Geometry: see drawing. Coordinates: mm, zero at the bounding-box minimum. Round coordinates to 2 decimals unless told otherwise and drop trailing zeros. Loops run counter-clockwise (first coordinate to the right, second up) from the corner with the lowest first, then second, coordinate; pieces in that order, holes last. Notation, with made-up numbers: (19.25, 0) - (52.25, 0) arc R19 cw to (52.25, 30) - close; hole circle Ø8 at (81, -33.75). An arc over 180 degrees is marked (long way). Use CSV: the item, a comma, the result in double quotes.
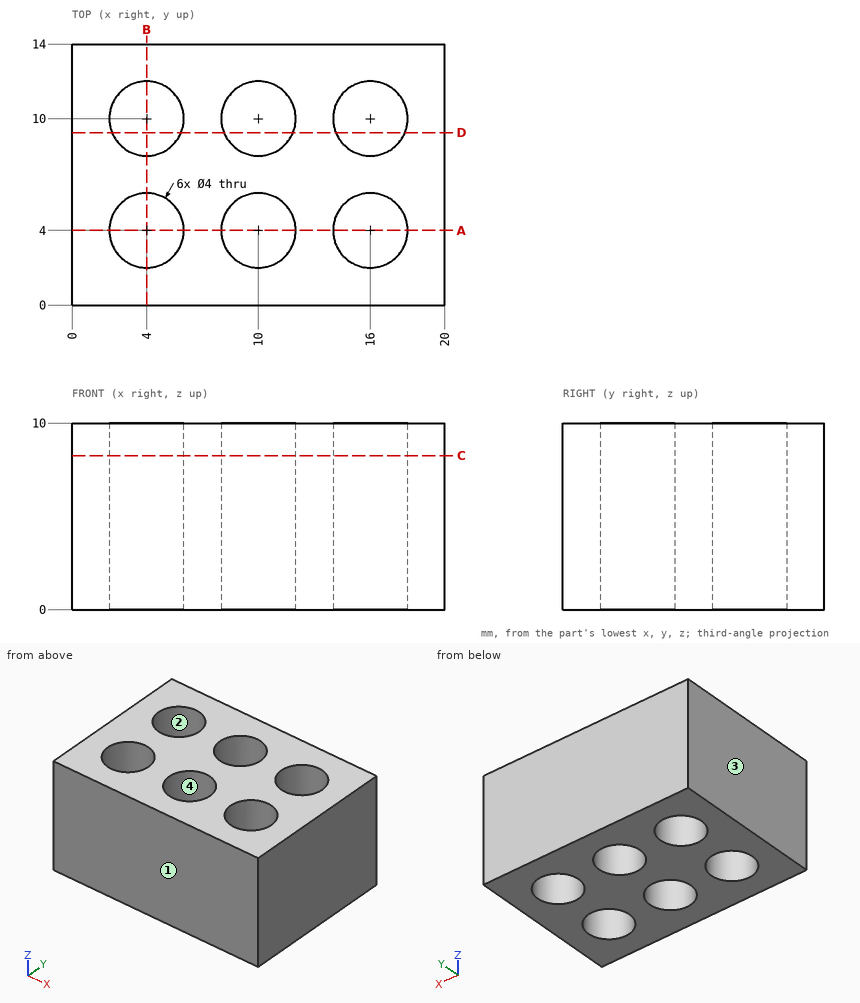
Item 1: Material intervals for line 1 (Y direction, x = 4, z = 6); line 2 (Y direction, x = 8.5, z = 7.25); line 3 (X direction, y = 4.75, z = 6.5), sorted ascending.
Final values:
line 1,"y = 0 to 2, 6 to 8, 12 to 14"
line 2,"y = 0 to 2.68, 5.32 to 8.68, 11.32 to 14"
line 3,"x = 0 to 2.15, 5.85 to 8.15, 11.85 to 14.15, 17.85 to 20"
Item 2: Mould query, pull axis Y, two halves, no side actions, for the marked faces 1, 2, 3 and 4. Classes: released by +Y, released by -Y, zero draft, split by the parting line, or undercut.
Final values:
face 1,"released by -Y"
face 2,"undercut"
face 3,"zero draft"
face 4,"undercut"
Item 3: Section D-D on y = 9.25. Return the cut outline in (x, z), plus the area to 3 significant figures.
Final values:
outline,"(0, 0) - (2.15, 0) - (2.15, 10) - (0, 10) - close; (5.85, 0) - (8.15, 0) - (8.15, 10) - (5.85, 10) - close; (11.85, 0) - (14.15, 0) - (14.15, 10) - (11.85, 10) - close; (17.85, 0) - (20, 0) - (20, 10) - (17.85, 10) - close"
area,"88.8 mm²"
Item 4: Section C-C on z = 8.25. Return the cut outline in (x, y), plus the area to 3 significant figures.
Final values:
outline,"(0, 0) - (20, 0) - (20, 14) - (0, 14) - close; hole circle Ø4 at (4, 4); hole circle Ø4 at (4, 10); hole circle Ø4 at (10, 4); hole circle Ø4 at (10, 10); hole circle Ø4 at (16, 4); hole circle Ø4 at (16, 10)"
area,"205 mm²"
Item 5: Section A-A on y = 4. Return the cut outline in (x, z), plus the area to 3 significant figures.
Final values:
outline,"(0, 0) - (2, 0) - (2, 10) - (0, 10) - close; (6, 0) - (8, 0) - (8, 10) - (6, 10) - close; (12, 0) - (14, 0) - (14, 10) - (12, 10) - close; (18, 0) - (20, 0) - (20, 10) - (18, 10) - close"
area,"80.0 mm²"
Item 6: Section B-B on x = 4. Return the cut outline in (y, z), plus the area to 3 significant figures.
Final values:
outline,"(0, 0) - (2, 0) - (2, 10) - (0, 10) - close; (6, 0) - (8, 0) - (8, 10) - (6, 10) - close; (12, 0) - (14, 0) - (14, 10) - (12, 10) - close"
area,"60.0 mm²"
Item 7: Pin query (flat end, axial travel): P1, Ø6, axis at x = 11, y = 11, coming from the +Z side. Return the tip coordinate at first contact, or that it passes through.
Final values:
P1,"stops at z = 10"
